Verification items for this drawing (mm, ordinates from the low corner). A direction names the side the tool comes from. Coordinates: 2 decimals unless noted, no trailing zeros. Order: outer loops, then holes, each group sorted by start corner. A loop starts at its lowest first (then second) coordinate and runs counter-clockwise, first axis right, second up. Notation, with made-up numbers: M 57,19 L 64,19 A8 cw 64,30 Z; hole C 79.5,40.25 d1. An arc over 180 degrees is marked long. One line per item, written item: value. Start each with the question number.
1) Sectioned sample at C-C, the plane x = 21.5. Enter the section's corners in (y, z), then the cut area to 3 significant figures.
2) Sectioned sample at B-B, the plane y = 1. Enter the section's corners in (x, z), then the cut area to 3 significant figures.
3) Thickness scan on L1, parallel to X at y = 2, z = 9.25; L2, parallel to Y at x = 51.5, z = 5.25; L3, parallel to X at y = 7.25, z = 12. Record the ranges inside material, lowest first. Write a range as from..to.
4) Sectioned sample at D-D, the plane z = 11. Enter the section's corners in (x, y), then the cut area to 3 significant figures.
5) Draft check along X on the marked faces 1, 2 and 3. Enter one of: pulls with the +X half, pulls with the -X half, needs draft (parallel to the pull), parting line crosses it, or undercut.
6) Sectioned sample at A-A, the plane z = 3.75. Enter the section's corners in (x, y), then the cut area to 3 significant figures.
7) Access from +Z, -Z, +X, -X, +Y, -Y to the whole of each face (thin tool, end or side, straight path). Record for the marked faces 4 and 5.
8) Go/stop test with flat-tipped pins: P1, Ø1.5, axis at x = 9, z = 3.5, coming from the -Y side; P2, Ø3, axis at y = 7.5, z = 8, coming from the +X side. Record where each tip stops, or that it passes through.
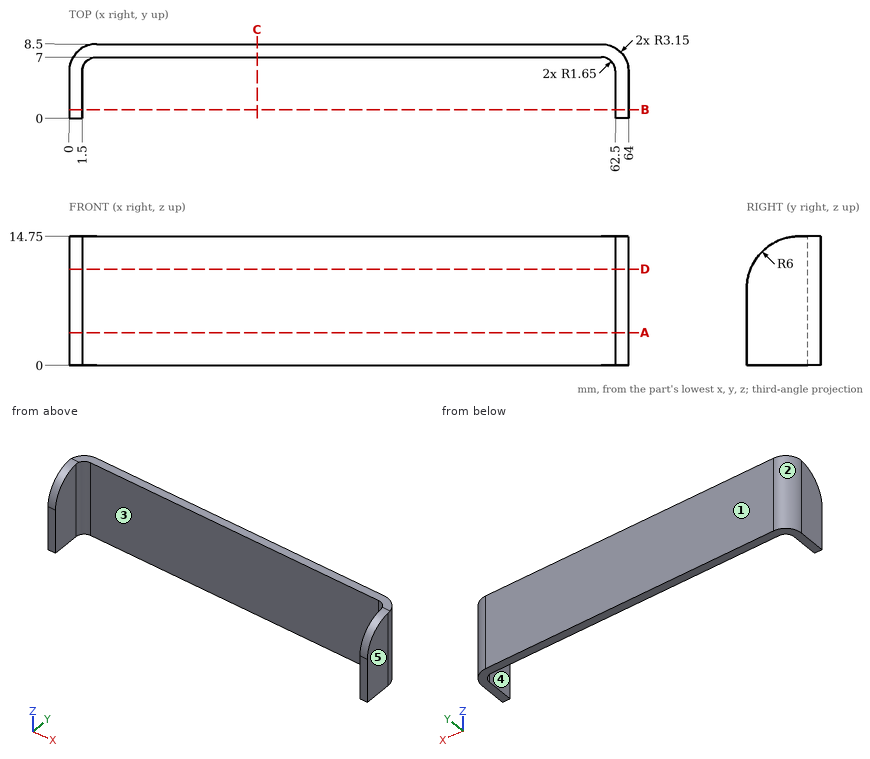
Final values:
1. outline: M 7,0 L 8.5,0 L 8.5,14.75 L 7,14.75 Z
1. area: 22.1 mm^2
2. outline: M 0,0 L 1.5,0 L 1.5,12.07 L 0,12.07 Z; M 62.5,0 L 64,0 L 64,12.07 L 62.5,12.07 Z
2. area: 36.2 mm^2
3. L1: x = 0..1.5, 62.5..64
3. L2: y = 7..8.5
3. L3: x = 0.64..63.36
4. outline: M 0,0.44 L 1.5,0.44 L 1.5,5.35 A1.65 cw 3.15,7 L 60.85,7 A1.65 cw 62.5,5.35 L 62.5,0.44 L 64,0.44 L 64,5.35 A3.15 ccw 60.85,8.5 L 3.15,8.5 A3.15 ccw 0,5.35 Z
4. area: 113 mm^2
5. face 1: needs draft
5. face 2: pulls with the -X half
5. face 3: undercut
6. outline: M 0,0 L 1.5,0 L 1.5,5.35 A1.65 cw 3.15,7 L 60.85,7 A1.65 cw 62.5,5.35 L 62.5,0 L 64,0 L 64,5.35 A3.15 ccw 60.85,8.5 L 3.15,8.5 A3.15 ccw 0,5.35 Z
6. area: 114 mm^2
7. face 4: +Z, -Z, -Y
7. face 5: +Z, -Z, +X, +Y, -Y
8. P1: stops at y = 7
8. P2: stops at x = 63.93
